Source: CAD feature listing. Evaluate the final solid. Frame: model axes, mm. A direction names the side the tool comes from. Round coordinates to 2 decimals unless told otherwise and drop trailing zeros. Write each loop counter-clockwise with the first axis right and the second up, starting at its lowest first coordinate (ties: lowest second). Pieces come first, ordered by that corner, then holes. Notation, with made-up numbers: (76.5, 85.25) -> (114.5, 85.25) arc R23 ccw to (114.5, 116.25) -> close; hole circle Ø10 at (74, 31). An arc over 180 degrees is marked (long way). Put each result on its own line as item: value.
Autodesk Inventor part; units mm, degrees
ref_plane "YZ Plane" through (0, 0, 0) normal (1, 0, 0) x (0, 1, 0)
ref_plane "XZ Plane" through (0, 0, 0) normal (0, 1, 0) x (-1, 0, 0)
ref_plane "XY Plane" through (0, 0, 0) normal (0, 0, 1) x (1, 0, 0)
sketch "Sketch1" plane through (0, 0, 0) normal (0, 0, 1) x (1, 0, 0)
  line L0 (0, 0) -> (0, 8)
  line L1 (0, 8) -> (7.8, 8)
  line L2 (7.8, 8) -> (7.8, 6)
  line L3 (7.8, 6) -> (14.8, 6)
  line L4 (14.8, 6) -> (14.8, 8)
  line L5 (14.8, 8) -> (16, 8)
  line L6 (16, 8) -> (16, 0)
  line L7 (16, 0) -> (0, 0)
  dimension "d0" = 16
  dimension "d1" = 1.2
  dimension "d2" = 7
  dimension "d3" = 16
  dimension "d4" = 12
revolve "Revolution1" add sketch "Sketch1" angle 360 about axis through (16, 0, 0) along (-1, 0, 0)
chamfer "Chamfer1" distance 0.2 angle 45 4 edges at (7.8, -8, 0) (0, -8, 0) (14.8, -8, 0) (16, -8, 0)
sketch "Sketch2" plane through (16, 0, 0) normal (1, 0, 0) x (0, 0, -1)
  circle A0 centre (0, 0) radius 2.5
  dimension "d9" = 5
extrude "Extrusion1" cut sketch "Sketch2" against normal through all
ref_plane "Work Plane1" through (8, 0, 0) normal (1, 0, 0) x (0, 0, -1)
properties part number "Riemenscheibe"
Q1. Material intervals for line 1 (Y direction, x = 6, z = 0); line 2 (Y direction, x = 12.75, z = 0); line 3 (X direction, y = -2.75, z = -6.25), sorted ascending. Write a range as [from, to].
Ans:
line 1: y = [-8, -2.5], [2.5, 8]
line 2: y = [-6, -2.5], [2.5, 6]
line 3: x = [0, 7.8], [14.8, 16]
Q2. Draft query along Z for faces 3 (the cylindrical face through (15.41, -1.73, -7.81)), 4 (the flat face through (0, -2, -2)), 5 (the cylindrical face through (8.11, -2.44, 0.54)). Return one class per face: +Z half, -Z half, draft (parallel to the pull), parting line (faces both ways), or undercut.
Ans:
face 3: parting line
face 4: draft
face 5: undercut
Q3. Cut plane C-C on x = 12.5. Output: boundary loops of the cut face in (y, z).
Ans:
outline: circle Ø12 at (0, 0); hole circle Ø5 at (0, 0)
Q4. Reachability of faces 1 (the flat face through (7.8, 4, 5)), 2 (the cylindrical face through (3.95, -1.73, -7.81)) from +Z, -Z, +X, -X, +Y, -Y: full face, straight path, thin tool, end or side. Return the list, or none.
Ans:
face 1: none
face 2: +X, -X
Q5. Cut plane D-D on x = 1.5. Output: boundary loops of the cut face in (y, z).
Ans:
outline: circle Ø16 at (0, 0); hole circle Ø5 at (0, 0)
Q6. Pin query (flat end, axial travel): pin 1 (4 mm diameter, centred on x = 10.5, y = -5, fed in from +Z); pin 2 (1 mm diameter, centred on x = 5, z = 2, fed in from +Y); pin 3 (1.5 mm diameter, centred on x = 9, y = -3, fed in from -Z). Return the tip coordinate at first contact, or that it passes through.
Ans:
pin 1: stops at z = 5.2
pin 2: stops at y = 7.86
pin 3: stops at z = -5.56
Q7. Cut plane A-A on y = 0. Output: boundary loops of the cut face in (x, z).
Ans:
outline: (0, -7.8) -> (0.2, -8) -> (7.6, -8) -> (7.8, -7.8) -> (7.8, -6) -> (14.8, -6) -> (14.8, -7.8) -> (15, -8) -> (15.8, -8) -> (16, -7.8) -> (16, -2.5) -> (0, -2.5) -> close; (0, 2.5) -> (16, 2.5) -> (16, 7.8) -> (15.8, 8) -> (15, 8) -> (14.8, 7.8) -> (14.8, 6) -> (7.8, 6) -> (7.8, 7.8) -> (7.6, 8) -> (0.2, 8) -> (0, 7.8) -> close
